The listing builds one solid part. Answer for the finished solid, in the listing's coordinates (mm). A direction names the side the tool comes from. Coordinates: 2 decimals unless noted, no trailing zeros. Loops run counter-clockwise (first coordinate to the right, second up) from the corner with the lowest first, then second, coordinate; pieces in that order, holes last. Notation, with made-up numbers: (55.25, -27.75) -> (101.25, -27.75) arc R20 cw to (101.25, -22.75) -> close; hole circle Ø7 at (25.5, -20). An arc over 180 degrees is marked (long way). Answer in a Markdown table with one row per item.
```python
from build123d import *

# Parameters (mm, degrees)
BOSS_EXTRUDE1_DEPTH = 8
SKETCH3_W           = 56.2
SKETCH3_H           = 30
BOSS_EXTRUDE2_DEPTH = 3
SKETCH4_R           = 1.7
SKETCH4_R_2         = 1.2
CUT_EXTRUDE2_DEPTH  = 11
CUT_EXTRUDE3_DEPTH  = 8
SKETCH7_R           = 2
SKETCH7_W           = 11.5
SKETCH7_H           = 5.4
CUT_EXTRUDE4_DEPTH  = 2
CUT_EXTRUDE6_REACH  = 13


with BuildPart() as part:
    # Sketch1 → Boss-Extrude1 (new body)
    with BuildSketch(Plane.XY):
        with BuildLine():
            Line((19.509889407, 0), (0, 0))
            Line((0, 0), (0, -30))
            Line((0, -30), (56.2, -30))
            Line((56.2, -30), (56.2, 0))
            Line((56.2, 0), (36.690110593, 0))
            Line((36.690110593, 0), (35.825930365, 0))
            ThreePointArc((35.825930365, 0), (34.325930365, -1.5), (35.825930365, -3))
            Line((35.825930365, -3), (37.988882647, -3))
            ThreePointArc((37.988882647, -3), (26.465465751, -15.568182447), (19.509889407, 0))
        make_face()
    extrude(amount=BOSS_EXTRUDE1_DEPTH)

    # Sketch3 → Boss-Extrude2 (add)
    with BuildSketch(Plane.XY.offset(8)):
        with Locations((28.1, -15)):
            Rectangle(SKETCH3_W, SKETCH3_H)
    extrude(amount=BOSS_EXTRUDE2_DEPTH)

    # Sketch4 → Cut-Extrude2 (cut)
    with BuildSketch(Plane(origin=(0, 0, 0), x_dir=(-1, 0, 0), z_dir=(0, 0, -1))):
        with Locations((-49.2, -7)):
            Circle(SKETCH4_R)
        with Locations((-7, -7)):
            Circle(SKETCH4_R)
        with Locations((-7, -23)):
            Circle(SKETCH4_R)
        with Locations((-49.2, -23)):
            Circle(SKETCH4_R)
        with Locations((-28.1, -5.5)):
            Circle(SKETCH4_R_2)
    extrude(amount=-CUT_EXTRUDE2_DEPTH, mode=Mode.SUBTRACT)

    # Sketch5 → Cut-Extrude3 (cut)
    with BuildSketch(Plane(origin=(0, 0, 0), x_dir=(-1, 0, 0), z_dir=(0, 0, -1))):
        with BuildLine():
            Line((-19.509889407, 0), (-36.690110593, 0))
            ThreePointArc((-36.690110593, 0), (-28.1, -15.7), (-19.509889407, 0))
        make_face()
    extrude(amount=-CUT_EXTRUDE3_DEPTH, mode=Mode.SUBTRACT)

    # Sketch7 → Cut-Extrude4 (cut)
    with BuildSketch(Plane.XY.offset(11)):
        with Locations((28.1, -5.5)):
            Circle(SKETCH7_R)
        with Locations((28.1, -10.7)):
            Rectangle(SKETCH7_W, SKETCH7_H)
    extrude(amount=-CUT_EXTRUDE4_DEPTH, mode=Mode.SUBTRACT)

    # Sketch9 → Cut-Extrude6 (cut, up to next)
    with BuildSketch(Plane.XY, mode=Mode.PRIVATE) as cut_extrude6_sk1:
        with BuildLine():
            Line((36.15, -30), (36.15, -17.197756195))
            ThreePointArc((36.15, -17.197756195), (28.1, -19.7), (20.05, -17.197756195))
            Line((20.05, -17.197756195), (20.05, -30))
            Line((20.05, -30), (36.15, -30))
        make_face()
    cut_extrude6_tool1 = extrude(cut_extrude6_sk1.sketch, amount=CUT_EXTRUDE6_REACH, mode=Mode.PRIVATE) & part.part
    add(cut_extrude6_tool1.solids().sort_by_distance((28.1, -24.424534, 0))[0], mode=Mode.SUBTRACT)


solid = part.part
```
Item 1: A cutting plane is placed at D-D, the plane y = -23.75. Determine the outline of the cut face in (x, z).
Findings below:
| item | result |
|---|---|
| outline | (0, 0) -> (5.47, 0) -> (5.47, 11) -> (0, 11) -> close; (8.53, 0) -> (20.05, 0) -> (20.05, 11) -> (8.53, 11) -> close; (36.15, 0) -> (47.67, 0) -> (47.67, 11) -> (36.15, 11) -> close; (50.73, 0) -> (56.2, 0) -> (56.2, 11) -> (50.73, 11) -> close |
Item 2: A cutting plane is placed at C-C, the plane z = 6. Determine the outline of the cut face in (x, y).
Findings below:
| item | result |
|---|---|
| outline | (0, -30) -> (20.05, -30) -> (20.05, -17.2) arc R14.2 ccw to (36.15, -17.2) -> (36.15, -30) -> (56.2, -30) -> (56.2, 0) -> (36.69, 0) arc R10.2 cw (long way) to (19.51, 0) -> (0, 0) -> close; hole circle Ø3.4 at (7, -23); hole circle Ø3.4 at (7, -7); hole circle Ø3.4 at (49.2, -23); hole circle Ø3.4 at (49.2, -7) |
Item 3: A cutting plane is placed at B-B, the plane y = -18.5. Determine the outline of the cut face in (x, z), plus the area to 3 significant figures.
Findings below:
| item | result |
|---|---|
| outline | (0, 0) -> (20.05, 0) -> (20.05, 11) -> (0, 11) -> close; (22.39, 0) -> (33.81, 0) -> (33.81, 11) -> (22.39, 11) -> close; (36.15, 0) -> (56.2, 0) -> (56.2, 11) -> (36.15, 11) -> close |
| area | 567 mm2 |
Item 4: Find the intervals of material crossed by probe 1 along Y at (x, z) = (7, 9.5); probe 2 along Y at (x, z) = (26.5, 9.25); probe 3 along X at (y, z) = (-23.25, 4.75), in increasing order.
Findings below:
| item | result |
|---|---|
| probe 1 | y = -30 to -24.7, -21.3 to -8.7, -5.3 to 0 |
| probe 2 | y = -19.61 to -13.4, -8 to -6.7, -4.3 to 0 |
| probe 3 | x = 0 to 5.32, 8.68 to 20.05, 36.15 to 47.52, 50.88 to 56.2 |
Item 5: A tool of negligible diameter and unlimited length cuts with its end or side. For faces 1 (the face through (28, -8, 10)), 2 (the face through (28, 0, 9)), 3 (the face through (36.15, -24, 5)), from which of +Z, -Z, +X, -X, +Y, -Y can it reach the whole face along a straight path? Write none if from no direction.
Findings below:
| item | result |
|---|---|
| face 1 | +Z |
| face 2 | +Z, -Z, +X, -X, +Y |
| face 3 | +Z, -Z, -Y |
Item 6: Flat-ended cylindrical pins translate along their axes: pin 1 Ø1.6 at (x, y) = (27, -10) entering from +Z; pin 2 Ø4.5 at (x, y) = (28.1, -5.5) entering from -Z; pin 3 Ø2.5 at (x, y) = (49.2, -7) entering from +Z; pin 4 Ø1.5 at (x, z) = (26.5, 1.5) entering from +Y. Find the tip coordinate at first contact, or state that the pin passes through.
Findings below:
| item | result |
|---|---|
| pin 1 | stops at z = 9 |
| pin 2 | stops at z = 8 |
| pin 3 | passes through |
| pin 4 | stops at y = -15.43 |
Item 7: Determine the mould class of faces 4 (the face through (28, -15, 11)), 5 (the face through (28.2, -19.7, 5.4)), 6 (the face through (0, -15, 5)) for opening direction X: +X half, -X half, draft (parallel to the pull), parting line (faces both ways), or undercut.
Findings below:
| item | result |
|---|---|
| face 4 | draft |
| face 5 | undercut |
| face 6 | -X half |
Item 8: A cutting plane is placed at A-A, the plane x = 7. Determine the outline of the cut face in (y, z), plus the area to 3 significant figures.
Findings below:
| item | result |
|---|---|
| outline | (-30, 0) -> (-24.7, 0) -> (-24.7, 11) -> (-30, 11) -> close; (-21.3, 0) -> (-8.7, 0) -> (-8.7, 11) -> (-21.3, 11) -> close; (-5.3, 0) -> (0, 0) -> (0, 11) -> (-5.3, 11) -> close |
| area | 255 mm2 |
